Here's how the part is built. I have some questions about the finished solid (model axes, mm). A direction names the side the tool comes from. Coordinates: 2 decimals unless noted, no trailing zeros. Write each loop counter-clockwise with the first axis right and the second up, starting at its lowest first coordinate (ties: lowest second). Pieces come first, ordered by that corner, then holes. Notation, with made-up numbers: (48.25, -9) -> (104.25, -9) arc R9 cw to (104.25, 6) -> close; hole circle Ø7 at (72, -27). An arc over 180 degrees is marked (long way). Use CSV: the item, a comma, the result in double quotes. Start each with the question number.
```python
from build123d import *

# Parameters (mm, degrees)
SKETCH1_TURRETBODYPARENT_11_W   = 1.5
SKETCH1_TURRETBODYPARENT_11_H   = 1.5
SKETCH1_TURRETBODYPARENT_11_W_2 = 22
SKETCH1_TURRETBODYPARENT_11_H_2 = 25
BOSS_EXTRUDE1_DEPTH             = 1.5
SKETCH1_TURRETBODYPARENT_13_W   = 22
SKETCH1_TURRETBODYPARENT_13_H   = 1.5
SKETCH1_TURRETBODYPARENT_13_W_2 = 1.5
SKETCH1_TURRETBODYPARENT_13_H_2 = 25
BOSS_EXTRUDE2_DEPTH             = 1.5


with BuildPart() as part:
    # Sketch1-turretBodyParent_11 → Boss-Extrude1 (new body)
    with BuildSketch(Plane(origin=(0, 0, 0), x_dir=(1, 0, 0), z_dir=(0, 1, 0))):
        Polygon((25, 28), (25, 25), (26.5, 25), (26.5, 29.5), (22, 29.5), (22, 28), align=None)
        Polygon((23.5, 26.5), (23.5, 25), (25, 25), (25, 28), (22, 28), (22, 26.5), align=None)
        with Locations((22.75, 25.75)):
            Rectangle(SKETCH1_TURRETBODYPARENT_11_W, SKETCH1_TURRETBODYPARENT_11_H)
        with Locations((11, 25.75)):
            Rectangle(SKETCH1_TURRETBODYPARENT_11_W_2, SKETCH1_TURRETBODYPARENT_11_H)
        with Locations((11, 27.25)):
            Rectangle(SKETCH1_TURRETBODYPARENT_11_W_2, SKETCH1_TURRETBODYPARENT_11_H)
        with Locations((11, 28.75)):
            Rectangle(SKETCH1_TURRETBODYPARENT_11_W_2, SKETCH1_TURRETBODYPARENT_11_H)
        Polygon((-4.5, 25), (-3, 25), (-3, 28), (0, 28), (0, 29.5), (-4.5, 29.5), align=None)
        Polygon((-3, 25), (-1.5, 25), (-1.5, 26.5), (0, 26.5), (0, 28), (-3, 28), align=None)
        with Locations((-0.75, 25.75)):
            Rectangle(SKETCH1_TURRETBODYPARENT_11_W, SKETCH1_TURRETBODYPARENT_11_H)
        with Locations((-0.75, 12.5)):
            Rectangle(SKETCH1_TURRETBODYPARENT_11_W, SKETCH1_TURRETBODYPARENT_11_H_2)
        with Locations((-2.25, 12.5)):
            Rectangle(SKETCH1_TURRETBODYPARENT_11_W, SKETCH1_TURRETBODYPARENT_11_H_2)
        with Locations((-3.75, 12.5)):
            Rectangle(SKETCH1_TURRETBODYPARENT_11_W, SKETCH1_TURRETBODYPARENT_11_H_2)
        with Locations((-0.75, -0.75)):
            Rectangle(SKETCH1_TURRETBODYPARENT_11_W, SKETCH1_TURRETBODYPARENT_11_H)
        Polygon((-1.5, -1.5), (-1.5, 0), (-3, 0), (-3, -3), (0, -3), (0, -1.5), align=None)
        Polygon((-3, -3), (-3, 0), (-4.5, 0), (-4.5, -4.5), (0, -4.5), (0, -3), align=None)
        with Locations((11, -3.75)):
            Rectangle(SKETCH1_TURRETBODYPARENT_11_W_2, SKETCH1_TURRETBODYPARENT_11_H)
        with Locations((11, -2.25)):
            Rectangle(SKETCH1_TURRETBODYPARENT_11_W_2, SKETCH1_TURRETBODYPARENT_11_H)
        Polygon((26.5, 0), (25, 0), (25, -3), (22, -3), (22, -4.5), (26.5, -4.5), align=None)
        Polygon((25, 0), (23.5, 0), (23.5, -1.5), (22, -1.5), (22, -3), (25, -3), align=None)
        with Locations((22.75, -0.75)):
            Rectangle(SKETCH1_TURRETBODYPARENT_11_W, SKETCH1_TURRETBODYPARENT_11_H)
        with Locations((22.75, 12.5)):
            Rectangle(SKETCH1_TURRETBODYPARENT_11_W, SKETCH1_TURRETBODYPARENT_11_H_2)
        with Locations((25.75, 12.5)):
            Rectangle(SKETCH1_TURRETBODYPARENT_11_W, SKETCH1_TURRETBODYPARENT_11_H_2)
        with Locations((24.25, 12.5)):
            Rectangle(SKETCH1_TURRETBODYPARENT_11_W, SKETCH1_TURRETBODYPARENT_11_H_2)
        with Locations((11, 12.5)):
            Rectangle(SKETCH1_TURRETBODYPARENT_11_W_2, SKETCH1_TURRETBODYPARENT_11_H_2)
        with Locations((11, -0.75)):
            Rectangle(SKETCH1_TURRETBODYPARENT_11_W_2, SKETCH1_TURRETBODYPARENT_11_H)
    extrude(amount=-BOSS_EXTRUDE1_DEPTH)

    # Sketch1-turretBodyParent_13 → Boss-Extrude2 (add)
    with BuildSketch(Plane(origin=(0, 0, 0), x_dir=(1, 0, 0), z_dir=(0, 1, 0))):
        Polygon((-4.5, 25), (-3, 25), (-3, 28), (0, 28), (0, 29.5), (-4.5, 29.5), align=None)
        with Locations((11, 28.75)):
            Rectangle(SKETCH1_TURRETBODYPARENT_13_W, SKETCH1_TURRETBODYPARENT_13_H)
        Polygon((25, 28), (25, 25), (26.5, 25), (26.5, 29.5), (22, 29.5), (22, 28), align=None)
        with Locations((25.75, 12.5)):
            Rectangle(SKETCH1_TURRETBODYPARENT_13_W_2, SKETCH1_TURRETBODYPARENT_13_H_2)
        Polygon((26.5, 0), (25, 0), (25, -3), (22, -3), (22, -4.5), (26.5, -4.5), align=None)
        with Locations((11, -3.75)):
            Rectangle(SKETCH1_TURRETBODYPARENT_13_W, SKETCH1_TURRETBODYPARENT_13_H)
        Polygon((-3, -3), (-3, 0), (-4.5, 0), (-4.5, -4.5), (0, -4.5), (0, -3), align=None)
        with Locations((-3.75, 12.5)):
            Rectangle(SKETCH1_TURRETBODYPARENT_13_W_2, SKETCH1_TURRETBODYPARENT_13_H_2)
        with Locations((-0.75, 25.75)):
            Rectangle(SKETCH1_TURRETBODYPARENT_13_W_2, SKETCH1_TURRETBODYPARENT_13_H)
        with Locations((11, 12.5)):
            Rectangle(SKETCH1_TURRETBODYPARENT_13_W, SKETCH1_TURRETBODYPARENT_13_H_2)
        with Locations((11, 25.75)):
            Rectangle(SKETCH1_TURRETBODYPARENT_13_W, SKETCH1_TURRETBODYPARENT_13_H)
        with Locations((22.75, 25.75)):
            Rectangle(SKETCH1_TURRETBODYPARENT_13_W_2, SKETCH1_TURRETBODYPARENT_13_H)
        with Locations((22.75, 12.5)):
            Rectangle(SKETCH1_TURRETBODYPARENT_13_W_2, SKETCH1_TURRETBODYPARENT_13_H_2)
        with Locations((22.75, -0.75)):
            Rectangle(SKETCH1_TURRETBODYPARENT_13_W_2, SKETCH1_TURRETBODYPARENT_13_H)
        with Locations((11, -0.75)):
            Rectangle(SKETCH1_TURRETBODYPARENT_13_W, SKETCH1_TURRETBODYPARENT_13_H)
        with Locations((-0.75, -0.75)):
            Rectangle(SKETCH1_TURRETBODYPARENT_13_W_2, SKETCH1_TURRETBODYPARENT_13_H)
        with Locations((-0.75, 12.5)):
            Rectangle(SKETCH1_TURRETBODYPARENT_13_W_2, SKETCH1_TURRETBODYPARENT_13_H_2)
    extrude(amount=BOSS_EXTRUDE2_DEPTH)


solid = part.part
```
Item 1: If I drill on line 1 along X through (y, z) = (1, -9); line 2 along Z through (x, y) = (10, 1.2); line 3 along Y through (x, z) = (-2, -13.5), over which ranges is the centre line in solid material (lowest first)?
Item 2: Thinking about a two-plate mould opening in X: for faces 1 (the flat face through (-4.5, 0, -13)), 2 (the flat face through (26.5, 0, -12)), 3 (the flat face through (-1.5, 1, -13)), which applies, +X half, -X half, draft (parallel to the pull), parting line (faces both ways), or undercut?
Item 3: Which directions (+Z, -Z, +X, -X, +Y, -Y) give clear straight access to the entire face, cutting with the end or side of a thin tool? Please do faces 4 (the flat face through (25, 1, -13)), 5 (the flat face through (11, 0, 4.5)).
Item 4: I want a section at B-B on x = 24. Please give me the cut outline in (y, z), then the cut area to 3 significant figures.
Item 5: I want a section at C-C on z = -8.5. Please give me the cut outline in (x, y), then the cut area to 3 significant figures.
Item 6: I want a section at A-A on y = 0.5. Please give me the cut outline in (x, z).
Geometry says:
1,line 1,"-4.5 to -3, -1.5 to 23.5, 25 to 26.5"
1,line 2,"-29.5 to -28, -26.5 to 1.5, 3 to 4.5"
1,line 3,"-1.5 to 0"
2,face 1,"-X half"
2,face 2,"+X half"
2,face 3,"undercut"
3,face 4,"+Y"
3,face 5,"+Z, +X, -X, +Y, -Y"
4,outline,"(-1.5, -29.5) -> (1.5, -29.5) -> (1.5, -28) -> (0, -28) -> (0, 3) -> (1.5, 3) -> (1.5, 4.5) -> (-1.5, 4.5) -> close"
4,area,"55.5 mm2"
5,outline,"(-4.5, -1.5) -> (26.5, -1.5) -> (26.5, 1.5) -> (25, 1.5) -> (25, 0) -> (23.5, 0) -> (23.5, 1.5) -> (-1.5, 1.5) -> (-1.5, 0) -> (-3, 0) -> (-3, 1.5) -> (-4.5, 1.5) -> close"
5,area,"88.5 mm2"
6,outline,"(-4.5, -29.5) -> (26.5, -29.5) -> (26.5, 4.5) -> (-4.5, 4.5) -> close; (-1.5, -26.5) -> (23.5, -26.5) -> (23.5, 1.5) -> (-1.5, 1.5) -> close; hole (-3, -28) -> (25, -28) -> (25, 3) -> (-3, 3) -> close"
